Build history of the part. All positions in model axes, mm. A direction names the side the tool comes from. Coordinates: 2 decimals unless noted, no trailing zeros. Loops run counter-clockwise (first coordinate to the right, second up) from the corner with the lowest first, then second, coordinate; pieces in that order, holes last. Notation, with made-up numbers: (38, 47.5) - (81, 47.5) arc R35 ccw to (81, 83.5) - close; hole circle Ø4 at (28, 63). An arc over 180 degrees is marked (long way). One line per item, written item: value.
```python
from build123d import *

# Parameters (mm, degrees)
BOSS_EXTRUDE1_DEPTH = 4.826
SKETCH3_R           = 3.72872
CUT_EXTRUDE1_DEPTH  = 0.9652
CHAMFER1_SIZE       = 1
CHAMFER1_SIZE2      = 1.732050808


with BuildPart() as part:
    # Sketch1 → Revolve1 (revolve)
    with BuildSketch(Plane.XY, mode=Mode.PRIVATE) as revolve1_sk:
        Polygon((4.6228, 6.096), (3.8608, 6.096), (3.8608, 4.6609), (-0.9652, 4.6609), (-0.9652, 0), (0, 0), (4.6228, 0), (23.6728, 0), (23.6728, 3.175), (4.6228, 3.175), align=None)
    revolve(revolve1_sk.sketch.rotate(Axis((4.6228, 0, 0), (1, 0, 0)), 180), axis=Axis((4.6228, 0, 0), (1, 0, 0)))

    # Sketch2 → Boss-Extrude1 (add)
    with BuildSketch(Plane.ZY.offset(-3.8608)):
        Polygon((0, 5.381943739), (-4.6609, 2.69097187), (-4.6609, -2.69097187), (0, -5.381943739), (4.6609, -2.69097187), (4.6609, 2.69097187), align=None)
    extrude(amount=BOSS_EXTRUDE1_DEPTH)

    # Sketch3 → Cut-Extrude1 (cut)
    with BuildSketch(Plane.ZY.offset(0.9652)):
        with Locations(Location((0, 0, 0), (0, 0, 270))):
            Circle(SKETCH3_R)
    extrude(amount=-CUT_EXTRUDE1_DEPTH, mode=Mode.SUBTRACT)

    # Chamfer1
    chamfer1_edges = [part.edges().sort_by_distance(p)[0] for p in [
        (23.6728, 3.175, 0),
    ]]
    chamfer1_side = [part.faces().sort_by_distance(p)[0] for p in [
        (23.6728, 0, 0),
    ]]
    chamfer(chamfer1_edges, length=CHAMFER1_SIZE, length2=CHAMFER1_SIZE2, reference=chamfer1_side[0])


solid = part.part
```
Item 1: Cut at A-A, the plane y = 0. Write the cut outline in (x, z) (3 decimals).
Check result:
outline: (-0.965, -4.661) - (3.861, -4.661) - (3.861, -6.096) - (4.623, -6.096) - (4.623, -3.175) - (21.941, -3.175) - (23.673, -2.175) - (23.673, 2.175) - (21.941, 3.175) - (4.623, 3.175) - (4.623, 6.096) - (3.861, 6.096) - (3.861, 4.661) - (-0.965, 4.661) - (-0.965, 3.729) - (0, 3.729) - (0, -3.729) - (-0.965, -3.729) - close
Item 2: Tool access for faces 4 (the face through (0, 0, 0)), 5 (the face through (1.482, -4.055, 2.298)), 6 (the face through (1.48, -4.02, -2.36)), 7 (the face through (1.48, 4.02, 2.36)), 8 (the face through (1, 0, -4.661)): list every direction of +Z, -Z, +X, -X, +Y, -Y with a clear straight run to the whole face (end or side of a thin tool).
Check result:
face 4: -X
face 5: +Z, -X, -Y
face 6: -Z, -X, -Y
face 7: +Z, -X, +Y
face 8: -Z, -X, +Y, -Y
Item 3: Pull direction Y, two halves, no side cores. Call faces 1 (the face through (1, 0, 4.661)), 2 (the face through (-0.49, 0.81, -3.64)), 3 (the face through (1.482, 4.055, -2.298)): released by +Y, released by -Y, zero draft, split by the parting line, or undercut.
Check result:
face 1: zero draft
face 2: undercut
face 3: released by +Y
Item 4: Cut at D-D, the plane y = 4. Write the cut outline in (x, z).
Check result:
outline: (-0.97, -2.39) - (3.86, -2.39) - (3.86, -4.6) - (4.62, -4.6) - (4.62, 4.6) - (3.86, 4.6) - (3.86, 2.39) - (-0.97, 2.39) - close
Item 5: Cut at C-C, the plane x = 2. Write the cut outline in (y, z).
Check result:
outline: (-5.38, 0) - (-2.69, -4.66) - (2.69, -4.66) - (5.38, 0) - (2.69, 4.66) - (-2.69, 4.66) - close
Item 6: Drop flat-ended pins along their axis: P1, Ø2, axis at y = 0.5, z = -4.5, coming from the +X side; P2, Ø5, axis at x = 2, z = 0.5, coming from the +Y side; P3, Ø2, axis at y = 0, z = -1.5, coming from the -X side; P4, Ø1, axis at y = 3.5, z = 4.5, coming from the -X side. Give the stop position or say it passes through.
Check result:
P1: stops at x = 4.62
P2: stops at y = 6.1
P3: stops at x = 0
P4: stops at x = 3.86
Item 7: Probe probe 1 along Z at (x, y) = (-0.7, 0); probe 2 along X at (y, z) = (-2.25, 3.5); probe 3 along X at (y, z) = (2.5, 5). List the from-to ranges inside material, lowest first. Write a range as from..to.
Check result:
probe 1: z = -4.66..-3.73, 3.73..4.66
probe 2: x = -0.97..4.62
probe 3: x = 3.86..4.62
Item 8: Cut at B-B, the plane z = 4. Write the cut outline in (x, y).
Check result:
outline: (-0.97, -3.07) - (3.86, -3.07) - (3.86, -4.6) - (4.62, -4.6) - (4.62, 4.6) - (3.86, 4.6) - (3.86, 3.07) - (-0.97, 3.07) - close
